Print and shaded views of the part. All mm, measured from the part's lowest x, y and z. Coordinates: 2 decimals unless noted, no trailing zeros. Order: outer loops, then holes, each group sorted by start corner. A loop starts at its lowest first (then second) coordinate and runs counter-clockwise, first axis right, second up.
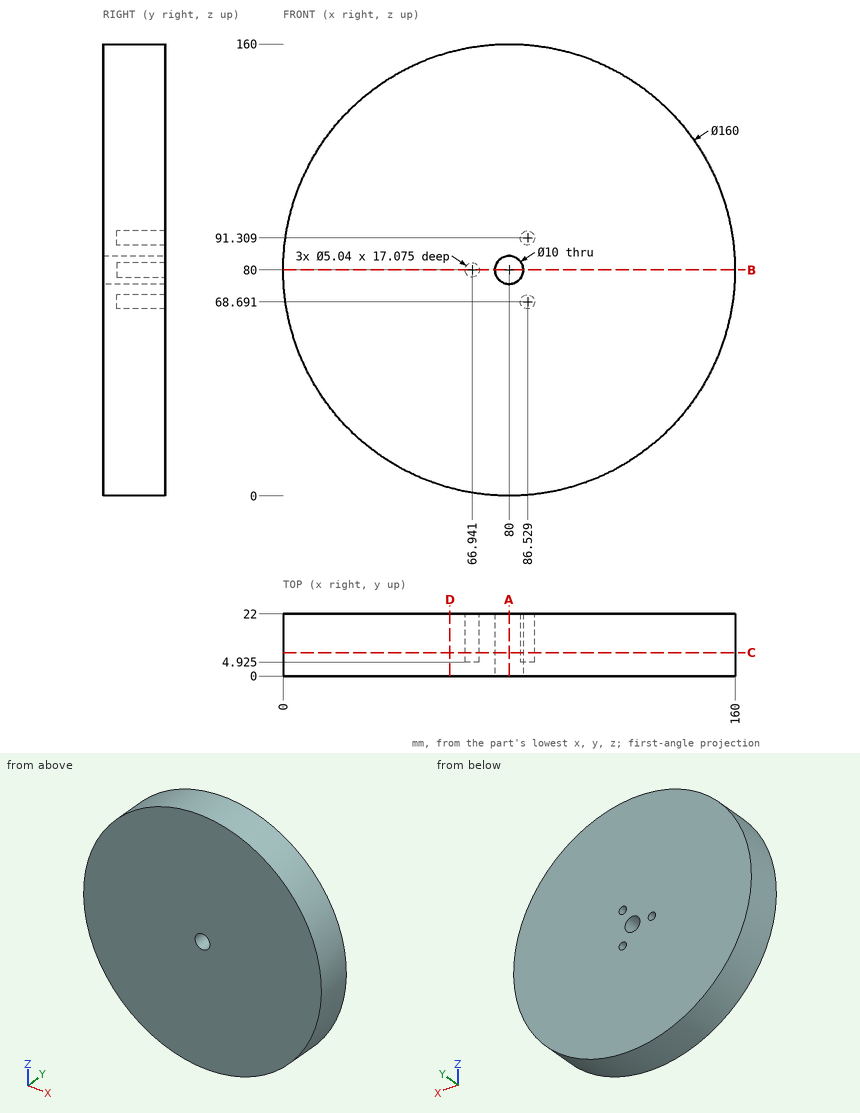
Q1. Cut at D-D, the plane x = 59. List the corners of the cut face in (y, z) (1 decimal).
Established:
outline: (0, 2.8) - (22, 2.8) - (22, 157.2) - (0, 157.2) - close
Q2. Cut at B-B, the plane z = 80. List the corners of the cut face in (x, y) (1 decimal), plus the area to 3 significant figures.
Established:
outline: (0, 0) - (75, 0) - (75, 22) - (69.5, 22) - (69.5, 4.9) - (64.4, 4.9) - (64.4, 22) - (0, 22) - close; (85, 0) - (160, 0) - (160, 22) - (85, 22) - close
area: 3,210 mm2
Q3. Cut at A-A, the plane x = 80. List the corners of the cut face in (y, z).
Established:
outline: (0, 0) - (22, 0) - (22, 75) - (0, 75) - close; (0, 85) - (22, 85) - (22, 160) - (0, 160) - close
Q4. Cut at C-C, the plane y = 8.25. List the corners of the cut face in (x, z), plus the area to 3 significant figures.
Established:
outline: circle Ø160 at (80, 80); hole circle Ø5.04 at (66.94, 80); hole circle Ø10 at (80, 80); hole circle Ø5.04 at (86.53, 68.69); hole circle Ø5.04 at (86.53, 91.31)
area: 20,000 mm2
Q5. Drop flat-ended pins along their axis: P1, Ø3, axis at y = 16.5, z = 128.5, coming from the +X side; P2, Ø1.5, axis at x = 67, z = 79.5, coming from the +Y side (1 decimal); P3, Ø6, axis at x = 80, z = 80, coming from the +Y side; P4, Ø5, axis at x = 32, y = 14, coming from the -Z side. Give the stop position or say it passes through.
Established:
P1: stops at x = 144.74
P2: stops at y = 4.9
P3: passes through
P4: stops at z = 14.2
Q6. Probe line 1 (X direction, y = 16.5, z = 80); line 2 (Z direction, x = 149, y = 2.75) (1 decimal); line 3 (X direction, y = 14.25, z = 143) (1 decimal). List the from-to ranges inside material, lowest first.
Established:
line 1: x = 0 to 64.42, 69.46 to 75, 85 to 160
line 2: z = 39.5 to 120.5
line 3: x = 30.7 to 129.3
